Solid Edge part; units mm, degrees
sketch "Sketch1" plane through (0, 0, 0) normal (0, -1, 0) x (1, 0, 0)
  line L0 (18.45, -2) -> (18.45, -12)
  line L1 (18.45, -12) -> (36.8105, -12)
  line L2 (36.8105, -12) -> (36.8105, 8.183)
  line L3 (36.8105, 8.183) -> (26.633, 8.183)
  line L4 (26.633, 8.183) -> (19.8642, 1.4142)
  line L5 (19.8642, 1.4142) -> (18.45, -2)
extrude "Protrusion1" add sketch "Sketch1" against normal blind 40
sketch "Sketch2" plane through (18.45, 20, -5.3442) normal (-1, 0, 0) x (0, -1, 0)
  line L0 (16.2229, -1.4749) -> (15, -0.2085)
  line L1 (15, -0.2085) -> (13.7771, -1.4749)
  arc A0 (13.7771, -1.4749) -> (16.2229, -1.4749) centre (15, -2.6558) ccw
  line L2 (-16.2229, -1.4749) -> (-15, -0.2085)
  line L3 (-15, -0.2085) -> (-13.7771, -1.4749)
  arc A1 (-13.7771, -1.4749) -> (-16.2229, -1.4749) centre (-15, -2.6558) cw
extrude "Cutout1" cut sketch "Sketch2" against normal up to next
sketch "Sketch3" plane through (23.5609, 20, 5.1109) normal (-0.7071, 0, 0.7071) x (0.7071, 0, 0.7071)
  line L0 (-0.4746, -9.2229) -> (0.7918, -8)
  line L1 (0.7918, -8) -> (-0.4746, -6.7771)
  arc A0 (-0.4746, -6.7771) -> (-0.4746, -9.2229) centre (-1.6555, -8) ccw
  line L2 (-0.4746, 9.2229) -> (0.7918, 8)
  line L3 (0.7918, 8) -> (-0.4746, 6.7771)
  arc A1 (-0.4746, 6.7771) -> (-0.4746, 9.2229) centre (-1.6555, 8) cw
extrude "ExtrudedCutout_2" cut sketch "Sketch3" against normal blind 30
sketch "Sketch4" plane through (32.7412, 20, 8.183) normal (0, 0, 1) x (0, 1, 0)
  circle A0 centre (-8, 0.0447) radius 1.7
  circle A1 centre (8, 0.0447) radius 1.7
extrude "Cutout2" cut sketch "Sketch4" against normal through all
sketch "Sketch5" plane through (29.8265, 40, -2.4295) normal (0, 1, 0) x (1, 0, 0)
  line L0 (-3.5071, 9.5705) -> (6.984, 9.5705)
  line L1 (6.984, 9.5705) -> (6.984, -0.9206)
  line L2 (6.984, -0.9206) -> (-3.5071, 9.5705)
extrude "ExtrudedCutout_5" cut sketch "Sketch5" against normal blind 40
sketch "Sketch6" plane through (31.7217, 20, 8.183) normal (0, 0, 1) x (0, 1, 0)
  circle A0 centre (15, -1.0888) radius 1.7
  circle A1 centre (-15, -1.0888) radius 1.7
extrude "ExtrudedCutout_11" cut sketch "Sketch6" against normal blind 22
sketch "Sketch7" plane through (31.7217, 20, 5.183) normal (0, 0, 1) x (-1, 0, 0)
  line L0 (-10.8423, -17.75) -> (1.0752, -17.75)
  line L1 (1.0752, -17.75) -> (2.6629, -15)
  line L2 (2.6629, -15) -> (1.0752, -12.25)
  line L3 (1.0752, -12.25) -> (-10.8423, -12.25)
  line L4 (-10.8423, -12.25) -> (-10.8423, -17.75)
  line L5 (-10.8423, 17.75) -> (1.0752, 17.75)
  line L6 (1.0752, 17.75) -> (2.6629, 15)
  line L7 (2.6629, 15) -> (1.0752, 12.25)
  line L8 (1.0752, 12.25) -> (-10.8423, 12.25)
  line L9 (-10.8423, 12.25) -> (-10.8423, 17.75)
  dimension "D1" = 10.8423
extrude "ExtrudedCutout_12" cut sketch "Sketch7" against normal blind 2.7
sketch "Sketch8" plane through (21.45, 20, -7) normal (-1, 0, 0) x (0, -1, 0)
  line L0 (-17.75, 1.1626) -> (-17.75, -12.7107)
  line L1 (-17.75, -12.7107) -> (-12.25, -12.7107)
  line L2 (-12.25, -12.7107) -> (-12.25, 1.1626)
  line L3 (-15, 4.0103) -> (-12.25, 1.1626)
  line L4 (-17.75, 1.1626) -> (-15, 4.0103)
  line L5 (17.75, 1.1626) -> (17.75, -12.7107)
  line L6 (17.75, -12.7107) -> (12.25, -12.7107)
  line L7 (12.25, -12.7107) -> (12.25, 1.1626)
  line L8 (15, 4.0103) -> (12.25, 1.1626)
  line L9 (17.75, 1.1626) -> (15, 4.0103)
  dimension "D1" = 17.75
  dimension "D2" = 17.75
extrude "ExtrudedCutout_13" cut sketch "Sketch8" against normal blind 3
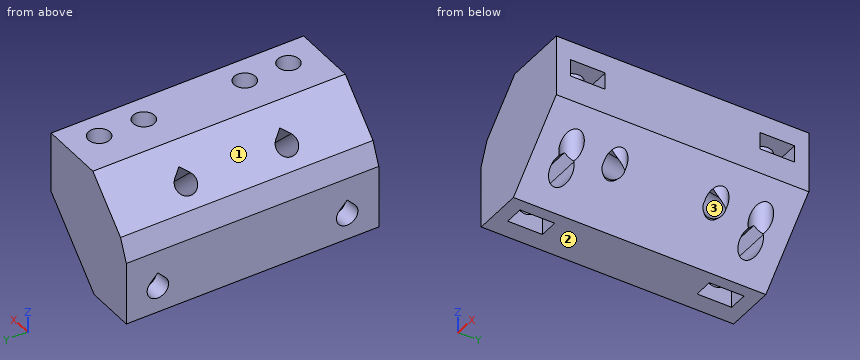
Work out the finished part from the listing and answer in its coordinate system (mm). Face numbers are marked on the shaded views. Round coordinates to 2 decimals unless told otherwise and drop trailing zeros. Loops run counter-clockwise (first coordinate to the right, second up) from the corner with the lowest first, then second, coordinate; pieces in that order, holes last. Notation, with made-up numbers: (45.25, 9) - (61.25, 9) arc R4 ccw to (61.25, 13) - close; hole circle Ø10 at (38.25, 66). An arc over 180 degrees is marked (long way). Use one line per item in the form item = value. Start each with the question number.
(1) Find section A-A on z = -8. Determine the outline of the cut face in (x, y), and give its area (3 significant figures).
(2) Flat-ended cylindrical pins translate along their axes: P1, Ø2, axis at x = 28.5, y = 17.5, coming from the -Z side; P2, Ø4.5, axis at y = 35.5, z = -5.5, coming from the +X side; P3, Ø2, axis at y = 15.5, z = 6, coming from the -X side; P4, Ø3, axis at y = 5, z = -8, coming from the +X side. Find the tip coordinate at first contact, or state that the pin passes through.
(3) Determine the mould class of the marked faces 1, 2 and 3 for opening direction X: +X half, -X half, draft (parallel to the pull), parting line (faces both ways), or undercut.
(4) Consider line 1 (Y direction, x = 19.8, z = -8); line 2 (Y direction, x = 23.25, z = -10.75); line 3 (Y direction, x = 31.75, z = 4). Determine where each line is inside the solid, lowest interval first.
(5) Find section D-D on x = 25.75. Give the number of separate pieces and of enclosed holes in the cut face, and give its area (3 significant figures).
(6) Find section B-B on y = 25. Determine the outline of the cut face in (x, z).
(7) Find section C-C on x = 35. Determine the outline of the cut face in (y, z), and give its area (3 significant figures).
Answer list:
q1.outline = (18.45, 0) - (30.32, 0) - (30.32, 3.3) - (24.45, 3.3) - (24.45, 2.25) - (21.45, 2.25) - (21.45, 3.3) - (18.45, 3.3) - close; (18.45, 6.7) - (21.45, 6.7) - (21.45, 7.75) - (24.45, 7.75) - (24.45, 6.7) - (30.32, 6.7) - (30.32, 33.3) - (24.45, 33.3) - (24.45, 32.25) - (21.45, 32.25) - (21.45, 33.3) - (18.45, 33.3) - close; (18.45, 36.7) - (21.45, 36.7) - (21.45, 37.75) - (24.45, 37.75) - (24.45, 36.7) - (30.32, 36.7) - (30.32, 40) - (18.45, 40) - close
q1.area = 381 mm^2
q2.P1 = -10.82
q2.P2 = 35.07
q2.P3 = 23.45
q2.P4 = through
q3.face_1 = -X half
q3.face_2 = draft
q3.face_3 = undercut
q4.line_1 = 0 to 3.3, 6.7 to 33.3, 36.7 to 40
q4.line_2 = 0 to 2.25, 7.75 to 32.25, 37.75 to 40
q4.line_3 = 0 to 2.25, 7.75 to 10.59, 13.41 to 26.59, 29.41 to 32.25, 37.75 to 40
q5.separate_pieces = 1
q5.enclosed_holes = 4
q5.area = 725 mm^2
q6.outline = (18.45, -12) - (26.32, -12) - (36.81, -1.51) - (36.81, 8.18) - (26.63, 8.18) - (19.86, 1.41) - (18.45, -2) - close
q7.outline = (0, -3.32) - (40, -3.32) - (40, 8.18) - (0, 8.18) - close; hole (2.25, 2.48) - (7.75, 2.48) - (7.75, 5.18) - (2.25, 5.18) - close; hole (32.25, 2.48) - (37.75, 2.48) - (37.75, 5.18) - (32.25, 5.18) - close
q7.area = 430 mm^2
